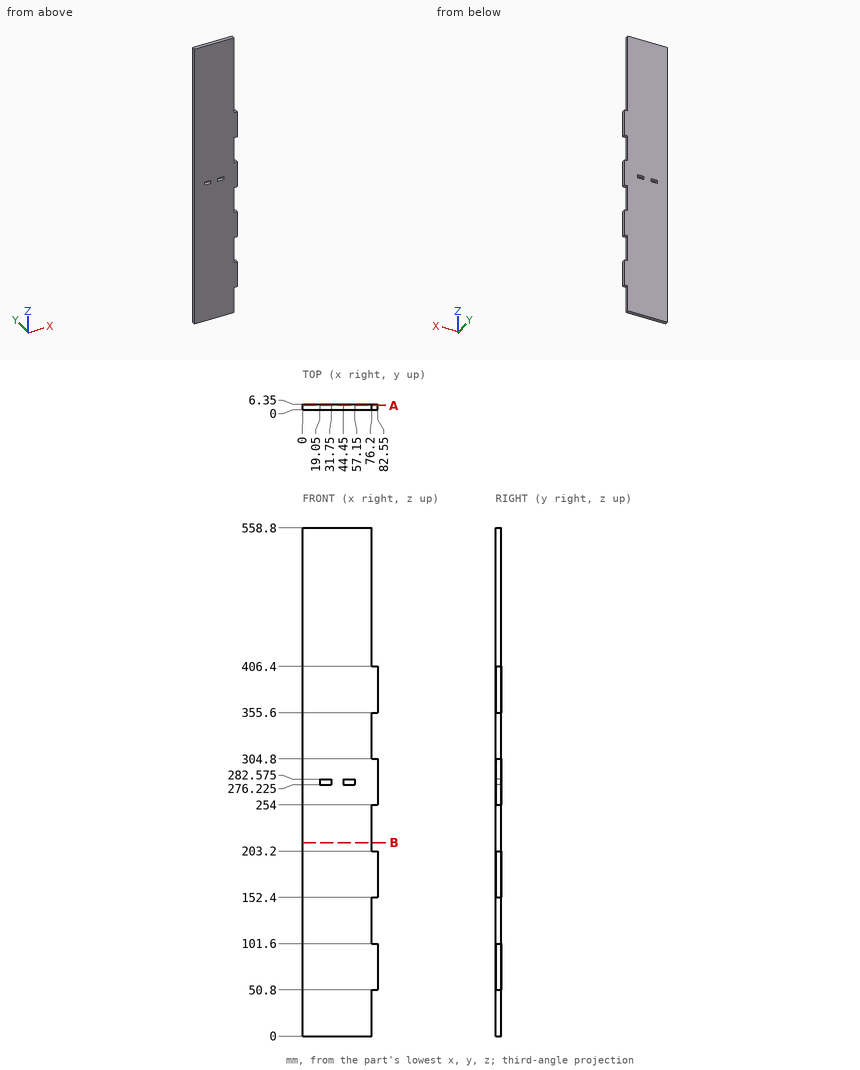
Answer from the drawing. Dimensions are ordinates in mm from the lowest x, y and z of the part. Coordinates: 2 decimals unless noted, no trailing zeros. Loops run counter-clockwise (first coordinate to the right, second up) from the corner with the lowest first, then second, coordinate; pieces in that order, holes last.
Q1. Each of these flat-tipped pins is pushed along its axis until it touches: pin 1 Ø1.9 at (x, y) = (80, 3.5) entering from -Z; pin 2 Ø2 at (y, z) = (3.5, 225.5) entering from +X; pin 3 Ø3 at (x, y) = (78.5, 4.5) entering from +Z. Where does it stop, or does it pass through?
Q2. Consider probe 1 along Z at (x, y) = (46, 5.25) (3 decimals); probe 2 along X at (y, z) = (1.5, 429.5). Determine where each line is inside the solid, lowest interval first.
Q3. The part is cut by section B-B on z = 212.5. Write down the section's boundary in (x, y), and give its area (3 significant figures).
Q4. The part is cut by section A-A on y = 4.75. Write down the section's boundary in (x, z) (3 decimals), and give its area (3 significant figures).
Results below:
1. pin 1: stops at z = 50.8
1. pin 2: stops at x = 76.2
1. pin 3: stops at z = 406.4
2. probe 1: z = 0 to 276.225, 282.575 to 558.8
2. probe 2: x = 0 to 76.2
3. outline: (0, 0) - (76.2, 0) - (76.2, 6.35) - (0, 6.35) - close
3. area: 484 mm2
4. outline: (0, 0) - (76.2, 0) - (76.2, 50.8) - (82.55, 50.8) - (82.55, 101.6) - (76.2, 101.6) - (76.2, 152.4) - (82.55, 152.4) - (82.55, 203.2) - (76.2, 203.2) - (76.2, 254) - (82.55, 254) - (82.55, 304.8) - (76.2, 304.8) - (76.2, 355.6) - (82.55, 355.6) - (82.55, 406.4) - (76.2, 406.4) - (76.2, 558.8) - (0, 558.8) - close; hole (19.05, 276.225) - (31.75, 276.225) - (31.75, 282.575) - (19.05, 282.575) - close; hole (44.45, 276.225) - (57.15, 276.225) - (57.15, 282.575) - (44.45, 282.575) - close
4. area: 43,700 mm2
